Model file for the job. Use its own axes, mm. A direction names the side the tool comes from. Round coordinates to 2 decimals unless told otherwise and drop trailing zeros. Write each loop counter-clockwise with the first axis right and the second up, starting at its lowest first coordinate (ties: lowest second). Pieces come first, ordered by that corner, then holes. Notation, with made-up numbers: (17, -9.75) - (43, -9.75) arc R23 cw to (43, 2.25) - close; hole circle Ø11 at (-3, 9). An arc over 180 degrees is marked (long way). Answer as a JSON object with one key per item and string values. Group by question number.
from build123d import *

# Parameters (mm, degrees)
SKETCH_1_R          = 18.5
EXTRUDE_1_DEPTH     = 6
SKETCH_6_R          = 13
EXTRUDE_2_DEPTH     = 6
SKETCH_8_R          = 2.5
SKETCH_8_R_2        = 2
CUT_EXTRUDE_1_DEPTH = 29.783675971


with BuildPart() as part:
    # Эскиз1 → Вытянуть1 (new body)
    with BuildSketch(Plane(origin=(0, 0, 0), x_dir=(1, 0, 0), z_dir=(0, 1, 0))):
        with Locations(Location((0, 0, 0), (0, 0, 270))):
            Circle(SKETCH_1_R)
    extrude(amount=EXTRUDE_1_DEPTH)

    # Вырез-По траектории1: sweep along a path in Эскиз3
    with BuildLine(Plane.XZ) as sweep_1_path:
        CenterArc((0, 0), 14.780391545, 0, 360)
    # Эскиз2 → Вырез-По траектории1 (sweep, cut)
    with BuildSketch(Plane.XY):
        with BuildLine():
            Line((-16.280391545, 0), (-13.280391545, 0))
            ThreePointArc((-13.280391545, 0), (-13.774210945, 0.666341341), (-14.533760145, 0.999438018))
            Line((-14.533760145, 0.999438018), (-15.027022944, 0.999438018))
            ThreePointArc((-15.027022944, 0.999438018), (-15.786572145, 0.666341341), (-16.280391545, 0))
        make_face()
    sweep(path=sweep_1_path.line, mode=Mode.SUBTRACT)

    # Вырез-По траектории2: sweep along a path in Эскиз5
    with BuildLine(Plane(origin=(0, 6, 0), x_dir=(1, 0, 0), z_dir=(0, 1, 0))) as sweep_2_path:
        CenterArc((0, 0), 15.352645825, 0, 360)
    # Эскиз4 → Вырез-По траектории2 (sweep, cut)
    with BuildSketch(Plane.XY):
        with BuildLine():
            Line((-16.751489622, 6), (-13.953802029, 6))
            ThreePointArc((-13.953802029, 6), (-14.416118652, 5.369797379), (-15.13270948, 5.05772433))
            Line((-15.13270948, 5.05772433), (-15.572582171, 5.05772433))
            ThreePointArc((-15.572582171, 5.05772433), (-16.289172999, 5.369797379), (-16.751489622, 6))
        make_face()
    sweep(path=sweep_2_path.line, mode=Mode.SUBTRACT)

    # Эскиз6 → Вытянуть2 (add)
    with BuildSketch(Plane(origin=(0, 6, 0), x_dir=(1, 0, 0), z_dir=(0, 1, 0))):
        with Locations(Location((0, 0, 0), (0, 0, 270))):
            Circle(SKETCH_6_R)
    extrude(amount=EXTRUDE_2_DEPTH)

    # Эскиз8 → Вырез-Вытянуть1 (cut, through all)
    with BuildSketch(Plane(origin=(0, 12, 0), x_dir=(1, 0, 0), z_dir=(0, 1, 0))):
        with Locations(Location((0, 0, 0), (0, 0, 270))):
            Circle(SKETCH_8_R)
        with Locations(Location((-3.894424366, -8.770838888, 0), (0, 0, 270))):
            Circle(SKETCH_8_R_2)
        with Locations(Location((8.770838888, -3.894424366, 0), (0, 0, 270))):
            Circle(SKETCH_8_R_2)
        with Locations(Location((3.894424366, 8.770838888, 0), (0, 0, 270))):
            Circle(SKETCH_8_R_2)
        with Locations(Location((-8.770838888, 3.894424366, 0), (0, 0, 270))):
            Circle(SKETCH_8_R_2)
    extrude(amount=-CUT_EXTRUDE_1_DEPTH, mode=Mode.SUBTRACT)


solid = part.part
(1) 3-axis set-ups, long thin cutter, end or side, ignore diameter. For faces 5 (the cylindrical face through (5.25, 6.08, -10.24)), 6 (the flat face through (12.5, 6, 4.1)): which of +Z, -Z, +X, -X, +Y, -Y reach the whole face in a straight line?
(2) Slice it at A-A (y = 10.5). Write the cut outline in (x, z).
(3) Drill centre lines: line 1 (X direction, y = 5.75, z = -9); line 2 (X direction, y = 1.5, z = 8.5); line 3 (Z direction, x = 4.5, y = 4.5). Where is each one in solid material? Low to high. Write a range as from..to.
(4) Pull direction Z, two halves, no side cores. Call faces 1 (the cylindrical face through (-7.91, 8.958, -10.316)), 2 (the cylindrical face through (-2.44, 6.08, -0.54)), 3 (the cylindrical face through (7, 6.08, 4.82)), 4 (the flat face through (-3, 12, 0)): pulls with the +Z half, pulls with the -Z half, needs draft (parallel to the pull), parting line crosses it, or undercut.
(5) Flat gauge pins, fed straight in: pin 1 (4 mm diameter, centred on y = 9.5, z = -11.5, fed in from +X); pin 2 (1.5 mm diameter, centred on y = 3.5, z = -10.5, fed in from +X). Where does each tip first touch, or does it go through?
Answer:
{
 "1": {"face 5": "+Y, -Y", "face 6": "+Y"},
 "2": {"outline": "circle Ø26 at (0, 0); hole circle Ø4 at (-8.77, -3.89); hole circle Ø4 at (-3.89, 8.77); hole circle Ø5 at (0, 0); hole circle Ø4 at (3.89, -8.77); hole circle Ø4 at (8.77, 3.89)"},
 "3": {"line 1": "-16.16..-13.98, -10.83..1.91, 5.88..10.83, 13.98..16.16", "line 2": "-16.43..-5.88, -1.91..16.43", "line 3": "-17.94..-10.68, -6.86..17.94"},
 "4": {"face 1": "parting line crosses it", "face 2": "undercut", "face 3": "undercut", "face 4": "needs draft"},
 "5": {"pin 1": "x = 8.87", "pin 2": "x = 15.72"}
}
